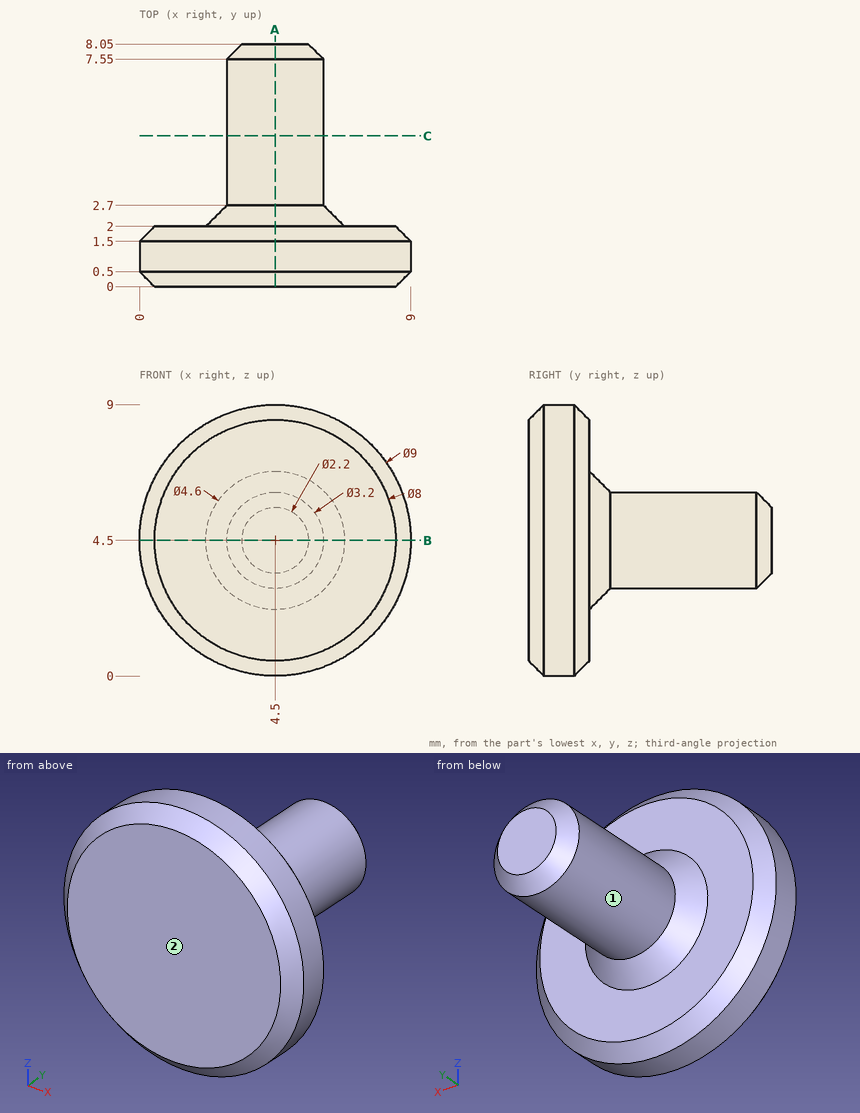
Geometry check sheet. Reference: drawing and pictorial views, mm from the part's lowest x, y, z. A direction names the side the tool comes from. Round coordinates to 2 decimals unless told otherwise and drop trailing zeros. Write each loop counter-clockwise with the first axis right and the second up, starting at its lowest first coordinate (ties: lowest second). Pieces come first, ordered by that corner, then holes.
Item 1: Section check A-A (x = 4.5). Record the boundary of the cut face in (y, z).
Determined:
outline: (0, 0.5) - (0.5, 0) - (1.5, 0) - (2, 0.5) - (2, 2.2) - (2.7, 2.9) - (7.55, 2.9) - (8.05, 3.4) - (8.05, 5.6) - (7.55, 6.1) - (2.7, 6.1) - (2, 6.8) - (2, 8.5) - (1.5, 9) - (0.5, 9) - (0, 8.5) - close
Item 2: Access from +Z, -Z, +X, -X, +Y, -Y to the whole of each face (thin tool, end or side, straight path). Record for the marked faces 1 and 2.
Determined:
face 1: +Y
face 2: +Z, -Z, +X, -X, -Y
Item 3: Material ranges on line 1 along Y through (x, z) = (6, 2.25); line 2 along Y through (x, z) = (2.75, 4.25); line 3 along Z through (x, y) = (4, 6.25), recorded low to high.
Determined:
line 1: y = 0 to 2
line 2: y = 0 to 2.53
line 3: z = 2.98 to 6.02
Item 4: Go/stop test with flat-tipped pins: pin 1 Ø4 at (y, z) = (2.5, 7) entering from +X; pin 2 Ø3 at (y, z) = (5, 6) entering from +X. Record where each tip stops, or that it passes through.
Determined:
pin 1: stops at x = 8.93
pin 2: stops at x = 6.1
Item 5: Section check C-C (y = 5). Record the boundary of the cut face in (x, z).
Determined:
outline: circle Ø3.2 at (4.5, 4.5)
Item 6: Section check B-B (z = 4.5). Record the boundary of the cut face in (x, y).
Determined:
outline: (0, 0.5) - (0.5, 0) - (8.5, 0) - (9, 0.5) - (9, 1.5) - (8.5, 2) - (6.8, 2) - (6.1, 2.7) - (6.1, 7.55) - (5.6, 8.05) - (3.4, 8.05) - (2.9, 7.55) - (2.9, 2.7) - (2.2, 2) - (0.5, 2) - (0, 1.5) - close
